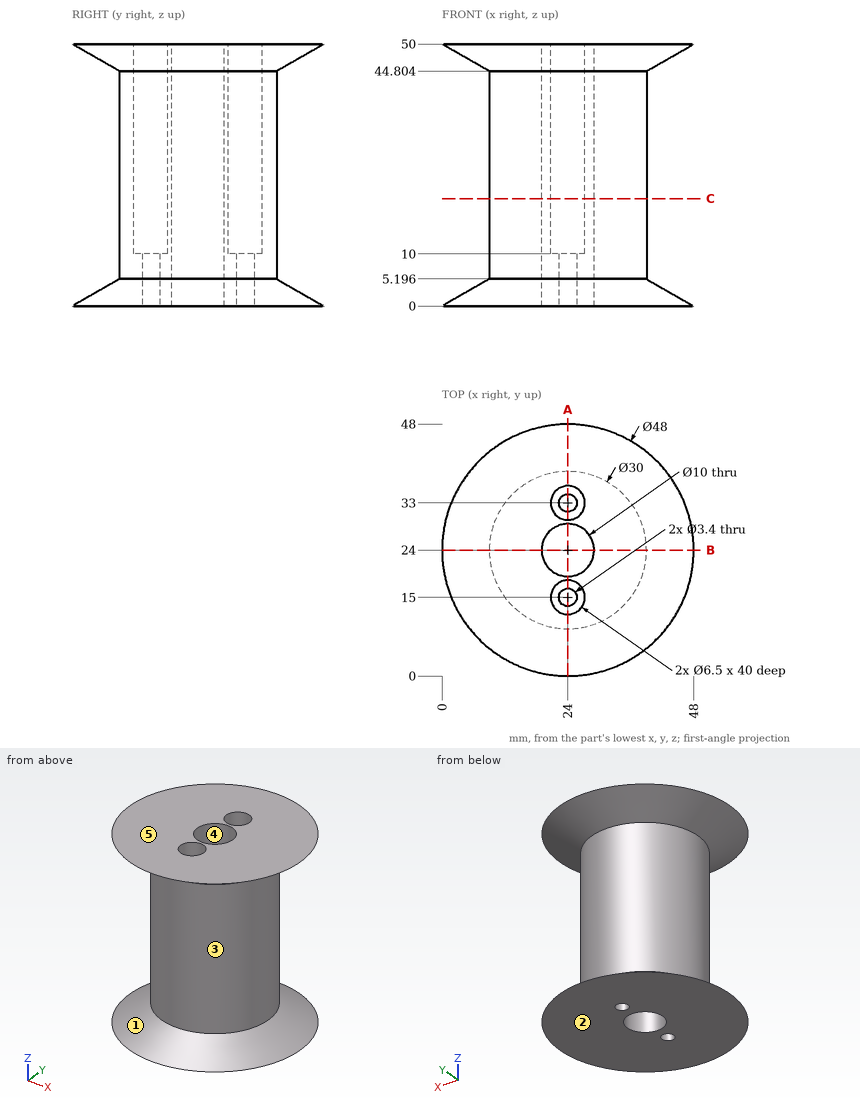
The figure shows three views and two pictorial views of one solid part (mm, origin at its lowest corner). Answer the questions. A direction names the side the tool comes from. Coordinates: 2 decimals unless noted, no trailing zeros. Loops run counter-clockwise (first coordinate to the right, second up) from the corner with the lowest first, then second, coordinate; pieces in that order, holes last. Notation, with made-up numbers: M 76.5,69 L 90.5,69 A25 ccw 90.5,82 Z; hole C -6,-34 d6. An arc over 180 degrees is marked long. Answer as CSV lines item,"result". Start each with the question number.
(1) Given pin 1 (2 mm diameter, centred on x = 22.5, y = 33, fed in from +Z); pin 2 (2 mm diameter, centred on x = 24, y = 26, fed in from -Z); pin 3 (12 mm diameter, centred on y = 30.5, z = 37.5, fed in from -X); pin 4 (1 mm diameter, centred on y = 14.5, z = 8, fed in from -X), each flat-ended and moving along its own axis, determine where each tip first touches the part or whether it passes through.
(2) For the marked faces 1 and 2, determine the directions among +Z, -Z, +X, -X, +Y, -Y from which every point of the face is accessible in a straight line to the end or side of a thin tool.
(3) The part is cut by section B-B (y = 24). Give the vertices of the cut face in (x, z).
(4) The mould has two halves that part along X. Classify the marked faces 3, 4 and 5: pulls with the +X half, pulls with the -X half, needs draft (parallel to the pull), parting line crosses it, or undercut.
(5) The part is cut by section A-A (x = 24). Give the vertices of the cut face in (y, z).
(6) The part is cut by section C-C (z = 20.5). Give the vertices of the cut face in (x, y), and give its area (3 significant figures).
(7) Find the intervals of material crossed by L1, parallel to X at y = 24, z = 13; L2, parallel to X at y = 24.5, z = 46 (1 decimal); L3, parallel to Z at x = 23, y = 4 (1 decimal), in increasing order. Write a range as [from, to].
Determined:
1,pin 1,"z = 10"
1,pin 2,"through"
1,pin 3,"x = 9.01"
1,pin 4,"x = 12"
2,face 1,"none"
2,face 2,"-Z, +X, -X, +Y, -Y"
3,outline,"M 0,0 L 19,0 L 19,50 L 0,50 L 9,44.8 L 9,5.2 Z; M 29,0 L 48,0 L 39,5.2 L 39,44.8 L 48,50 L 29,50 Z"
4,face 3,"parting line crosses it"
4,face 4,"undercut"
4,face 5,"needs draft"
5,outline,"M 0,0 L 13.3,0 L 13.3,10 L 11.75,10 L 11.75,50 L 0,50 L 9,44.8 L 9,5.2 Z; M 16.7,0 L 19,0 L 19,50 L 18.25,50 L 18.25,10 L 16.7,10 Z; M 29,0 L 31.3,0 L 31.3,10 L 29.75,10 L 29.75,50 L 29,50 Z; M 34.7,0 L 48,0 L 39,5.2 L 39,44.8 L 48,50 L 36.25,50 L 36.25,10 L 34.7,10 Z"
6,outline,"C 24,24 d30; hole C 24,24 d10; hole C 24,15 d6.5; hole C 24,33 d6.5"
6,area,"562 mm2"
7,L1,"[9, 19], [29, 39]"
7,L2,"[6.9, 19], [29, 41.1]"
7,L3,"[0, 2.3], [47.7, 50]"
